Part model, mm, in its own coordinate system. A direction names the side the tool comes from. Round coordinates to 2 decimals unless told otherwise and drop trailing zeros. Write each loop counter-clockwise with the first axis right and the second up, starting at its lowest first coordinate (ties: lowest second). Pieces come first, ordered by that corner, then holes. Notation, with made-up numbers: (38, 69) -> (57, 69) arc R8 cw to (57, 84) -> close; hole circle Ø8 at (60, 38). An arc over 180 degrees is marked (long way). Return JSON: item names as keys, results as strings. Group by question number.
(1) Tool access for faces 1 (the flat face through (0, -8.89, 0)), 2 (the flat face through (13, 6.223, 0)): list every direction of +Z, -Z, +X, -X, +Y, -Y with a clear straight run to the whole face (end or side of a thin tool).
(2) Saw through at A-A (x = 0). List the corners of the cut face in (y, z).
(3) Mould opens along Z. For faces 3 (the cylindrical face through (-13.97, 4.94, 0.06)), 4 (the flat face through (0, 60.833, 0)), 5 (the cylindrical face through (-0.34, -4.38, 1.55)) say: +Z half, -Z half, draft (parallel to the pull), parting line (faces both ways), or undercut.
(4) Drop flat-ended pins along their axis: pin 1 Ø3 at (x, z) = (-13, 0) entering from -Y; pin 2 Ø4 at (y, z) = (45, -3) entering from +X; pin 3 Ø1 at (y, z) = (24.5, 4.5) entering from -X. Give the stop position or say it passes through.
(5) Drill centre lines: L1, parallel to Y at x = -5.5, z = 0; L2, parallel to Y at x = -5.5, z = 7; L3, parallel to Z at x = 12.7, y = 5.35. Where is each one in solid material? Low to high. Write a range as from..to.
(6) Saw through at C-C (y = 44). List the corners of the cut face in (x, z), plus the area to 3 significant figures.
(7) Saw through at B-B (z = 0). List the corners of the cut face in (x, y).
(8) Saw through at D-D (x = 12.7). List the corners of the cut face in (y, z), plus the area to 3 significant figures.
Autodesk Inventor part; units mm, degrees
ref_plane "YZ Plane" through (0, 0, 0) normal (1, 0, 0) x (0, 1, 0)
ref_plane "XZ Plane" through (0, 0, 0) normal (0, 1, 0) x (-1, 0, 0)
ref_plane "XY Plane" through (0, 0, 0) normal (0, 0, 1) x (1, 0, 0)
sketch "Sketch1" plane through (0, 0, 0) normal (0, 1, 0) x (-1, 0, 0)
  circle A0 centre (0, 0) radius 6.5405
  dimension "d0" = 13.081
extrude "Extrusion1" add sketch "Sketch1" along normal blind 3.683
sketch "Sketch2" plane through (0, 3.683, 0) normal (0, 1, 0) x (1, 0, 0)
  circle A0 centre (0, 0) radius 19.05
  dimension "d3" = 38.1
extrude "Extrusion2" add sketch "Sketch2" along normal blind 57.15
sketch "Sketch3" plane through (0, 0, 0) normal (0, -1, 0) x (1, 0, 0)
  circle A0 centre (0, 0) radius 1.5875
  dimension "d6" = 3.175
extrude "Extrusion3" add sketch "Sketch3" along normal blind 8.89
sketch "Sketch4" plane through (0, 3.683, 0) normal (0, -1, 0) x (1, 0, 0)
  circle A0 centre (0, 0) radius 19.05
  circle A1 centre (0, 0) radius 12.7 construction
  circle A2 centre (0, 0) radius 1.5875
  line L0 (0, 0) -> (0, -12.7) construction
  line L1 (0, 0) -> (-12.7, 0) construction
  line L2 (0, 0) -> (12.7, 0) construction
  circle A3 centre (0, -12.7) radius 1.27
  circle A4 centre (-12.7, 0) radius 1.27
  circle A5 centre (12.7, 0) radius 1.27
  dimension "d9" = 25.4
  dimension "d10" = 2.54
extrude "Extrusion4" cut sketch "Sketch4" against normal blind 2.54 contours A3 | A4 | A5
properties part number "Motor"
Computed values:
{
 "1": {"face 1": "+Z, -Z, +X, -X, -Y", "face 2": "-Y"},
 "2": {"outline": "(-8.89, -1.59) -> (0, -1.59) -> (0, -6.54) -> (3.68, -6.54) -> (3.68, -11.43) -> (6.22, -11.43) -> (6.22, -13.97) -> (3.68, -13.97) -> (3.68, -19.05) -> (60.83, -19.05) -> (60.83, 19.05) -> (3.68, 19.05) -> (3.68, 6.54) -> (0, 6.54) -> (0, 1.59) -> (-8.89, 1.59) -> close"},
 "3": {"face 3": "undercut", "face 4": "draft", "face 5": "parting line"},
 "4": {"pin 1": "y = 3.68", "pin 2": "x = 19.02", "pin 3": "x = -18.63"},
 "5": {"L1": "0..60.83", "L2": "3.68..60.83", "L3": "-14.2..-1.27, 1.27..14.2"},
 "6": {"outline": "circle Ø38.1 at (0, 0)", "area": "1,140 mm2"},
 "7": {"outline": "(-19.05, 3.68) -> (-13.97, 3.68) -> (-13.97, 6.22) -> (-11.43, 6.22) -> (-11.43, 3.68) -> (-6.54, 3.68) -> (-6.54, 0) -> (-1.59, 0) -> (-1.59, -8.89) -> (1.59, -8.89) -> (1.59, 0) -> (6.54, 0) -> (6.54, 3.68) -> (11.43, 3.68) -> (11.43, 6.22) -> (13.97, 6.22) -> (13.97, 3.68) -> (19.05, 3.68) -> (19.05, 60.83) -> (-19.05, 60.83) -> close"},
 "8": {"outline": "(3.68, -14.2) -> (60.83, -14.2) -> (60.83, 14.2) -> (3.68, 14.2) -> (3.68, 1.27) -> (6.22, 1.27) -> (6.22, -1.27) -> (3.68, -1.27) -> close", "area": "1,620 mm2"}
}
